```python
from build123d import *

# Parameters (mm, degrees)
SK_BOARD_W   = 85
SK_BOARD_H   = 1.6
BOARD_DEPTH  = 28
SK_COOLER_W  = 40
SK_COOLER_H  = 10
COOLER_DEPTH = 20
SK_PORTS_W   = 17.5
SK_PORTS_H   = 16
PORTS_DEPTH  = 26.5


with BuildPart() as part:
    # SK_Board → Board (new, symmetric)
    with BuildSketch(Plane.XY):
        with Locations((0, 0.8)):
            Rectangle(SK_BOARD_W, SK_BOARD_H)
    extrude(amount=BOARD_DEPTH, both=True)

    # SK_Cooler → Cooler (add, symmetric)
    with BuildSketch(Plane.XY):
        with Locations((-5, 6.6)):
            Rectangle(SK_COOLER_W, SK_COOLER_H)
    extrude(amount=COOLER_DEPTH, both=True)

    # SK_Ports → Ports (add, symmetric)
    with BuildSketch(Plane.XY):
        with Locations((33.75, 9.6)):
            Rectangle(SK_PORTS_W, SK_PORTS_H)
    extrude(amount=PORTS_DEPTH, both=True)


solid = part.part
```
Work out the finished part from the listing and answer in its coordinate system (mm). A direction names the side the tool comes from. Round coordinates to 2 decimals unless told otherwise and drop trailing zeros. Loops run counter-clockwise (first coordinate to the right, second up) from the corner with the lowest first, then second, coordinate; pieces in that order, holes last. Notation, with made-up numbers: (14, 88) -> (40, 88) arc R32 cw to (40, 127) -> close; hole circle Ø11 at (-12.5, 33). An arc over 180 degrees is marked (long way). Write each question's results on one line, items separated by ' | '. Start each with the question number.
1. Section C-C (x = 30.5) is taken. Determine the outline of the cut face in (y, z).
2. Find the intervals of material crossed by probe 1 along X at (y, z) = (9.25, -17); probe 2 along X at (y, z) = (13.25, -13); probe 3 along Z at (x, y) = (30.5, 11.25), in increasing order. Write a range as from..to.
3. Section D-D (z = -23) is taken. Determine the outline of the cut face in (x, y).
4. A tool of negligible diameter and unlimited length cuts with its end or side. For faces 1 (the face through (15, 7, 0)), 2 (the face through (-5, 7, -20)), 3 (the face through (-5, 7, 20)), from which of +Z, -Z, +X, -X, +Y, -Y can it reach the whole face along a straight path? Write none if from no direction.
5. For a pull along X with two mould halves and no side action, classify faces 4 (the face through (-5, 11.6, 0)), 5 (the face through (42.5, 9, 0)), 6 (the face through (-29, 1.6, 0)) as +X half, -X half, draft (parallel to the pull), parting line (faces both ways), or undercut.
6. Given pin 1 Ø1.5 at (x, y) = (29, 6.5) entering from -Z; pin 2 Ø5 at (y, z) = (5.5, -12) entering from -X; pin 3 Ø1 at (x, y) = (-17.5, 13.5) entering from -Z; pin 4 Ø4 at (x, y) = (11.5, 13) entering from -Z, each flat-ended and moving along its own axis, determine where each tip first touches the part or whether it passes through.
7. Section A-A (y = 8.75) is taken. Determine the outline of the cut face in (x, z).
8. Section B-B (z = 8.5) is taken. Determine the outline of the cut face in (x, y).
Evaluation:
1) outline: (0, -28) -> (1.6, -28) -> (1.6, -26.5) -> (17.6, -26.5) -> (17.6, 26.5) -> (1.6, 26.5) -> (1.6, 28) -> (0, 28) -> close
2) probe 1: x = -25..15, 25..42.5 | probe 2: x = 25..42.5 | probe 3: z = -26.5..26.5
3) outline: (-42.5, 0) -> (42.5, 0) -> (42.5, 17.6) -> (25, 17.6) -> (25, 1.6) -> (-42.5, 1.6) -> close
4) face 1: +Z, -Z, +Y | face 2: -Z, -X, +Y | face 3: +Z, -X, +Y
5) face 4: draft | face 5: +X half | face 6: undercut
6) pin 1: stops at z = -26.5 | pin 2: stops at x = -25 | pin 3: passes through | pin 4: stops at z = -20
7) outline: (-25, -20) -> (15, -20) -> (15, 20) -> (-25, 20) -> close; (25, -26.5) -> (42.5, -26.5) -> (42.5, 26.5) -> (25, 26.5) -> close
8) outline: (-42.5, 0) -> (42.5, 0) -> (42.5, 17.6) -> (25, 17.6) -> (25, 1.6) -> (15, 1.6) -> (15, 11.6) -> (-25, 11.6) -> (-25, 1.6) -> (-42.5, 1.6) -> close
